Could you check a few things on this model? Use its own coordinates, in mm. A direction names the side the tool comes from. Give positions to 0.01 mm unless a question says otherwise; leave off trailing zeros. Write each loop counter-clockwise with the first axis right and the second up, starting at its lowest first coordinate (ties: lowest second). Pieces come first, ordered by that corner, then holes. Notation, with made-up numbers: (-6, 40.5) - (41, 40.5) arc R27 ccw to (41, 63.5) - close; hole circle Ø9 at (83, 39.5). An arc over 180 degrees is marked (long way). Answer in a Markdown table with one row per item.
from build123d import *

# Parameters (mm, degrees)
SKETCH1_R          = 32
BASE_FLANGE1_DEPTH = 1.5
SKETCH6_R          = 1.6
CUT_EXTRUDE1_DEPTH = 46.279686395
SKETCH7_R          = 4.8
SKETCH7_R_2        = 1.25
CUT_EXTRUDE2_DEPTH = 46.279686395
SKETCH9_W          = 9
SKETCH9_H          = 6
CUT_EXTRUDE3_DEPTH = 46.279686395
FILLET1_R          = 1


# Sheet-metal steps are written as plain solids
with BuildPart() as part:
    # Sketch1 → Base-Flange1 (new body)
    with BuildSketch(Plane(origin=(0, 0, 0), x_dir=(1, 0, 0), z_dir=(0, 1, 0))):
        with Locations(Location((0, 0, 0), (0, 0, 270))):
            Circle(SKETCH1_R)
    extrude(amount=-BASE_FLANGE1_DEPTH)

    # Sketch6 → Cut-Extrude1 (cut, through all)
    with BuildSketch(Plane(origin=(0, 0, 0), x_dir=(1, 0, 0), z_dir=(0, 1, 0))):
        with Locations(Location((0, -28, 0), (0, 0, 270))):
            Circle(SKETCH6_R)
        with Locations(Location((-24.248711306, 14, 0), (0, 0, 270))):
            Circle(SKETCH6_R)
        with Locations(Location((24.248711306, 14, 0), (0, 0, 270))):
            Circle(SKETCH6_R)
    extrude(amount=-CUT_EXTRUDE1_DEPTH, mode=Mode.SUBTRACT)

    # Sketch7 → Cut-Extrude2 (cut, through all)
    with BuildSketch(Plane(origin=(0, 0, 0), x_dir=(1, 0, 0), z_dir=(0, 1, 0))):
        with Locations(Location((0, 0, 0), (0, 0, 270))):
            Circle(SKETCH7_R)
        with Locations(Location((-4.949747468, 4.949747468, 0), (0, 0, 270))):
            Circle(SKETCH7_R_2)
        with Locations(Location((4.949747468, 4.949747468, 0), (0, 0, 270))):
            Circle(SKETCH7_R_2)
        with Locations(Location((4.949747468, -4.949747468, 0), (0, 0, 270))):
            Circle(SKETCH7_R_2)
        with Locations(Location((-4.949747468, -4.949747468, 0), (0, 0, 270))):
            Circle(SKETCH7_R_2)
    extrude(amount=-CUT_EXTRUDE2_DEPTH, mode=Mode.SUBTRACT)

    # Sketch9 → Cut-Extrude3 (cut, through all)
    with BuildSketch(Plane(origin=(0, 0, 0), x_dir=(1, 0, 0), z_dir=(0, 1, 0))):
        with Locations((0, -21)):
            Rectangle(SKETCH9_W, SKETCH9_H)
    extrude(amount=-CUT_EXTRUDE3_DEPTH, mode=Mode.SUBTRACT)

    # Fillet1
    fillet1_edges = [part.edges().sort_by_distance(p)[0] for p in [
        (-4.5, -0.75, 24),
        (-4.5, -0.75, 18),
        (4.5, -0.75, 18),
        (4.5, -0.75, 24),
    ]]
    fillet(fillet1_edges, radius=FILLET1_R)


solid = part.part
1) Imagine slicing it at A-A (x = 0). List the corners of the cut face in (y, z) for me, then the cut area to 3 significant figures.
Check values:
| item | result |
|---|---|
| outline | (-1.5, -32) - (0, -32) - (0, -4.8) - (-1.5, -4.8) - close; (-1.5, 4.8) - (0, 4.8) - (0, 18) - (-1.5, 18) - close; (-1.5, 24) - (0, 24) - (0, 26.4) - (-1.5, 26.4) - close; (-1.5, 29.6) - (0, 29.6) - (0, 32) - (-1.5, 32) - close |
| area | 67.8 mm2 |
2) If I drill on line 1 (Z direction, x = -6, y = -1.3); line 2 (X direction, y = -0.7, z = -14); line 3 (X direction, y = -0.75, z = 27), over which ranges is the centre line in solid material (lowest first)?
Check values:
| item | result |
|---|---|
| line 1 | z = -31.43 to -5.63, -4.27 to 4.27, 5.63 to 31.43 |
| line 2 | x = -28.77 to -25.85, -22.65 to 22.65, 25.85 to 28.77 |
| line 3 | x = -17.18 to -1.25, 1.25 to 17.18 |
3) On a 3-axis mill with a long thin cutter (end or side, diameter ignored), from which of +Z, -Z, +X, -X, +Y, -Y can I reach the whole of each face in a straight line? I mean faces 1 (the face through (0, -1, 18)), 2 (the face through (-7, 0, 0)). Say none if no direction works.
Check values:
| item | result |
|---|---|
| face 1 | +Y, -Y |
| face 2 | +Z, -Z, +X, -X, +Y |
4) Imagine slicing it at C-C (y = -1.05). State how many separate pieces and enclosed holes the cut face has, then the cut area to 3 significant figures.
Check values:
| item | result |
|---|---|
| separate pieces | 1 |
| enclosed holes | 9 |
| area | 3,050 mm2 |
5) Imagine slicing it at D-D (z = -14). List the corners of the cut face in (x, y) for me, then the cut area to 3 significant figures.
Check values:
| item | result |
|---|---|
| outline | (-28.77, -1.5) - (-25.85, -1.5) - (-25.85, 0) - (-28.77, 0) - close; (-22.65, -1.5) - (22.65, -1.5) - (22.65, 0) - (-22.65, 0) - close; (25.85, -1.5) - (28.77, -1.5) - (28.77, 0) - (25.85, 0) - close |
| area | 76.7 mm2 |
6) We'd pull the mould along Z, two halves only. Please class faces 3 (the face through (-7, -1.5, 0)), 4 (the face through (-24.2, -0.7, -15.6)), 5 (the face through (-31.24, -0.74, -6.94)): +Z half, -Z half, draft (parallel to the pull), parting line (faces both ways), or undercut.
Check values:
| item | result |
|---|---|
| face 3 | draft |
| face 4 | undercut |
| face 5 | parting line |
7) Imagine slicing it at B-B (z = 0). List the corners of the cut face in (x, y) for me, then the cut area to 3 significant figures.
Check values:
| item | result |
|---|---|
| outline | (-32, -1.5) - (-4.8, -1.5) - (-4.8, 0) - (-32, 0) - close; (4.8, -1.5) - (32, -1.5) - (32, 0) - (4.8, 0) - close |
| area | 81.6 mm2 |
8) Will these pins go through, and if not, where does the flat tip stop? P1, Ø7.5, axis at x = 0, z = 0, coming from the +Y side; P2, Ø0.8, axis at x = -1.5, y = -0.5, coming from the +Z side; P3, Ø0.8, axis at x = -1, y = -0.5, coming from the -Z side.
Check values:
| item | result |
|---|---|
| P1 | passes through |
| P2 | stops at z = 31.98 |
| P3 | stops at z = -31.99 |
